Print and shaded views of the part. All mm, measured from the part's lowest x, y and z. Round coordinates to 2 decimals unless told otherwise and drop trailing zeros. Write each loop counter-clockwise with the first axis right and the second up, starting at its lowest first coordinate (ties: lowest second). Pieces come first, ordered by that corner, then holes. Notation, with made-up numbers: (-0.5, 22) -> (19.5, 22) arc R19 ccw to (19.5, 59) -> close; hole circle Ø2 at (27.25, 55.25). An arc over 180 degrees is marked (long way). Return JSON: item names as keys, results as strings. Group by question number.
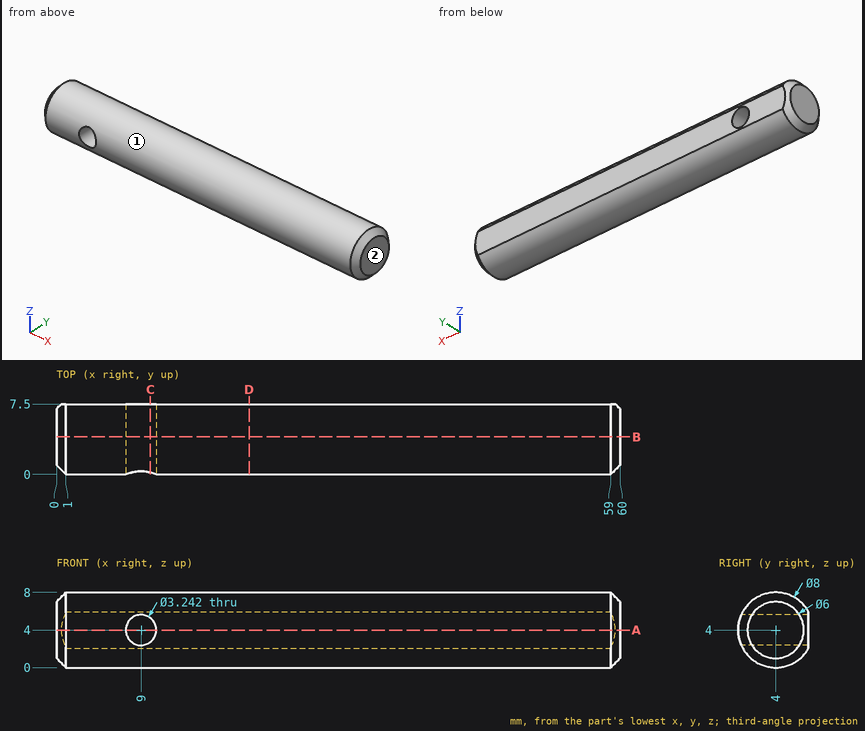
Item 1: Wall check: L1, parallel to Y at x = 21, z = 7.5; L2, parallel to Z at x = 9, y = 2; L3, parallel to Z at x = 9, y = 4.5. Give the ranges that are in metal, low to high.
Item 2: Cut at C-C (x = 10). Write the cut outline in (y, z), then the cut area to 3 significant figures.
Item 3: Cut at B-B (y = 4). Write the cut outline in (x, z).
Item 4: Two-plate mould, pull along Z, no slides. Class the marked faces 1 and 2: released by +Z, released by -Z, zero draft, split by the parting line, or undercut.
Item 5: Flat gauge pins, fed straight in: P1, Ø2, axis at x = 30, y = 1.5, coming from the +Z side; P2, Ø3, axis at y = 6, z = 4.5, coming from the -X side; P3, Ø3, axis at x = 9, z = 4, coming from the +Y side. Where does each tip first touch, or does it go through?
Item 6: Cut at D-D (x = 20.5). Write the cut outline in (y, z).
Item 7: Cut at A-A (z = 4). Write the cut outline in (x, y).
Checks:
{
 "1": {"L1": "y = 2.06 to 5.94", "L2": "z = 0.54 to 2.38, 5.62 to 7.46", "L3": "z = 0.03 to 2.38, 5.62 to 7.97"},
 "2": {"outline": "(0.21, 2.72) arc R4 ccw to (7.5, 2.06) -> (7.5, 2.72) -> close; (0.21, 5.28) -> (7.5, 5.28) -> (7.5, 5.94) arc R4 ccw to start", "area": "30.0 mm2"},
 "3": {"outline": "(0, 1) -> (1, 0) -> (59, 0) -> (60, 1) -> (60, 7) -> (59, 8) -> (1, 8) -> (0, 7) -> close; hole circle Ø3.24 at (9, 4)"},
 "4": {"face 1": "split by the parting line", "face 2": "zero draft"},
 "5": {"P1": "stops at z = 7.71", "P2": "stops at x = 0", "P3": "passes through"},
 "6": {"outline": "(7.5, 2.06) -> (7.5, 5.94) arc R4 ccw (long way) to start"},
 "7": {"outline": "(0, 1) -> (1, 0) -> (7.38, 0) -> (7.38, 7.5) -> (0.5, 7.5) -> (0, 7) -> close; (10.62, 0) -> (59, 0) -> (60, 1) -> (60, 7) -> (59.5, 7.5) -> (10.62, 7.5) -> close"}
}
